Autodesk Inventor part; units mm, degrees
ref_plane "YZ Plane" through (0, 0, 0) normal (1, 0, 0) x (0, 1, 0)
ref_plane "XZ Plane" through (0, 0, 0) normal (0, 1, 0) x (-1, 0, 0)
ref_plane "XY Plane" through (0, 0, 0) normal (0, 0, 1) x (1, 0, 0)
sketch "Sketch1" plane through (0, 0, 0) normal (0, 1, 0) x (-1, 0, 0)
  arc A0 (12.5208, -2.4451) -> (12.5208, 2.4451) centre (12, 0) ccw
  arc A1 (1.0417, 4.8903) -> (1.0417, -4.8903) centre (0, 0) ccw
  line L0 (1.0417, 4.8903) -> (12.5208, 2.4451)
  line L1 (12.5208, -2.4451) -> (1.0417, -4.8903)
  dimension "d0" = 2.5
  dimension "d1" = 5
  dimension "d2" = 12
extrude "Extrusion1" add sketch "Sketch1" along normal blind 4
sketch "Sketch3" plane through (0, 4, 0) normal (0, 1, 0) x (1, 0, 0)
  arc A0 (-12.5208, 2.4451) -> (-12.5208, -2.4451) centre (-12, 0) ccw
  point P0 (0, 0)
hole "Hole2" at (-12, 4, 0) direction (0, -1, 0) diameter 2.459 end through all
sketch "Sketch4" plane through (0, 4, 0) normal (0, 1, 0) x (1, 0, 0)
  arc A0 (-1.0417, -4.8903) -> (-1.0417, 4.8903) centre (0, 0) ccw
hole "Hole3" at (0, 4, 0) direction (0, -1, 0) diameter 5.9175 end through all
properties part number "214.1"
Input: part model. Units: mm. Frame: model coordinates. Give positions to 0.01 mm unless a question says otherwise; leave off trailing zeros. Loops run counter-clockwise (first coordinate to the right, second up) from the corner with the lowest first, then second, coordinate; pieces in that order, holes last. Notation, with made-up numbers: (33, 46.25) -> (63, 46.25) arc R21 cw to (63, 66.25) -> close; hole circle Ø8 at (48.5, 4.5). An arc over 180 degrees is marked (long way). Answer as a JSON object with one key per item and string values. Group by question number.
Item 1: Cut plane B-B, the plane x = 0. Return the cut outline in (y, z), and give its area (3 significant figures).
Item 2: Cut plane C-C, the plane y = 3.55. Return the cut outline in (x, z), and give its area (3 significant figures).
Item 3: Line query: probe 1 along X at (y, z) = (3.2, 0); probe 2 along Z at (x, y) = (0, 3.6); probe 3 along X at (y, z) = (3.65, 0.75). Output: solid intervals per line, ascending.
Item 4: Cut plane D-D, the plane z = 2.75. Return the cut outline in (x, y), and give its area (3 significant figures).
Item 5: Cut plane A-A, the plane z = 0. Return the cut outline in (x, y), and give its area (3 significant figures).
Item 6: Pin query (flat end, axial travel): P1, Ø1.5, axis at x = -7.5, y = 1, coming from the +Z side; P2, Ø2, axis at y = 2.5, z = 4, coming from the +X side; P3, Ø1.5, axis at x = -11.5, y = 1, coming from the +Z side; P4, Ø1, axis at y = 3, z = 0.5, coming from the -X side. Return the tip coordinate at first contact, or that it passes through.
Item 7: Pull-direction query (Z, two-part tool) for faces 1 (the flat face through (-6.701, 1.972, 3.685)), 2 (the flat face through (-6.86, 1.97, -3.65)), 3 (the cylindrical face through (-12.831, 1.972, -0.906)); classes: released by +Z, released by -Z, zero draft, split by the parting line, or undercut.
Checks:
{
 "1": {"outline": "(0, -5) -> (4, -5) -> (4, -2.96) -> (0, -2.96) -> close; (0, 2.96) -> (4, 2.96) -> (4, 5) -> (0, 5) -> close", "area": "16.3 mm²"},
 "2": {"outline": "(-12.52, -2.45) -> (-1.04, -4.89) arc R5 ccw (long way) to (-1.04, 4.89) -> (-12.52, 2.45) arc R2.5 ccw to start; hole circle Ø2.46 at (-12, 0); hole circle Ø5.92 at (0, 0)", "area": "109 mm²"},
 "3": {"probe 1": "x = -14.5 to -13.23, -10.77 to -2.96, 2.96 to 5", "probe 2": "z = -5 to -2.96, 2.96 to 5", "probe 3": "x = -14.38 to -12.97, -11.03 to -2.86, 2.86 to 4.94"},
 "4": {"outline": "(-11.09, 0) -> (-1.09, 0) -> (-1.09, 4) -> (-11.09, 4) -> close; (1.09, 0) -> (4.18, 0) -> (4.18, 4) -> (1.09, 4) -> close", "area": "52.3 mm²"},
 "5": {"outline": "(-14.5, 0) -> (-13.23, 0) -> (-13.23, 4) -> (-14.5, 4) -> close; (-10.77, 0) -> (-2.96, 0) -> (-2.96, 4) -> (-10.77, 4) -> close; (2.96, 0) -> (5, 0) -> (5, 4) -> (2.96, 4) -> close", "area": "44.5 mm²"},
 "6": {"P1": "stops at z = 3.67", "P2": "stops at x = 4", "P3": "stops at z = 2.82", "P4": "stops at x = -14.5"},
 "7": {"face 1": "released by +Z", "face 2": "released by -Z", "face 3": "undercut"}
}
